```python
from build123d import *

# Parameters (mm, degrees)
BOSS_EXTRU_1_DEPTH      = 3
ESQUISSE2_R             = 17
ENL_V_MAT_EXTRU_1_DEPTH = 3
CONG_1_R                = 10


with BuildPart() as part:
    # Esquisse1 → Boss.-Extru.1 (new body)
    with BuildSketch(Plane.XY):
        Polygon((0, 0), (0, 35), (-3, 35), (-3, 65), (0, 65), (0, 100), (35, 100), (35, 103), (65, 103), (65, 100), (100, 100), (100, 65), (103, 65), (103, 35), (100, 35), (100, 0), (65, 0), (65, -3), (35, -3), (35, 0), align=None)
    extrude(amount=BOSS_EXTRU_1_DEPTH)

    # Esquisse2 → Enlèv. mat.-Extru.1 (cut)
    with BuildSketch(Plane.XY.offset(3)):
        with Locations((50, 50)):
            Circle(ESQUISSE2_R)
    extrude(amount=-ENL_V_MAT_EXTRU_1_DEPTH, mode=Mode.SUBTRACT)

    # Congé1
    cong_1_edges = [part.edges().sort_by_distance(p)[0] for p in [
        (0, 0, 1.5),
        (0, 100, 1.5),
        (100, 100, 1.5),
        (100, 0, 1.5),
    ]]
    fillet(cong_1_edges, radius=CONG_1_R)


solid = part.part
```
Model file for the job. Use its own axes, mm. A direction names the side the tool comes from. Coordinates: 2 decimals unless noted, no trailing zeros. Order: outer loops, then holes, each group sorted by start corner. A loop starts at its lowest first (then second) coordinate and runs counter-clockwise, first axis right, second up. Notation, with made-up numbers: (-25.5, 83.25) -> (-8.5, 83.25) arc R26 ccw to (-8.5, 103.25) -> close; hole circle Ø6 at (25.5, -16.5). An arc over 180 degrees is marked (long way). Answer as a JSON object with one key per item and string values. Group by question number.
1) Which spindle directions (+Z, -Z, +X, -X, +Y, -Y) get a long thin tool onto all of the face, cutting with end or side? Do faces 5 (the face through (65, -1, 1)), 6 (the face through (50, 103, 1)), 7 (the face through (100, 78, 1)), 8 (the face through (35, -2, 1)). Say none if no direction does.
2) Pull direction X, two halves, no side cores. Call faces 1 (the face through (46.315, 33.404, 1.521)), 2 (the face through (2.85, 3.01, 1.52)), 3 (the face through (77, 100, 1)), 4 (the face through (96.99, 97.15, 1.52)): +X half, -X half, draft (parallel to the pull), parting line (faces both ways), or undercut.
3) Cut at D-D, the plane y = 85. Write the cut outline in (x, z), then the cut area to 3 significant figures.
4) Cut at A-A, the plane x = 50. Write the cut outline in (y, z).
5) Drill centre lines: L1, parallel to Y at x = 50, z = 1.9; L2, parallel to Y at x = 42, z = 1; L3, parallel to X at y = 41, z = 2.7. Where is each one in solid material? Low to high.
6) Flat gauge pins, fed straight in: pin 1 (1.5 mm diameter, centred on x = 47.5, y = 34, fed in from -Z); pin 2 (1.5 mm diameter, centred on y = 23, z = 1, fed in from +X); pin 3 (1.5 mm diameter, centred on x = -1, z = 1, fed in from +Y). Where does each tip first touch, or does it go through?
7) Cut at C-C, the plane z = 1.6. Write the cut outline in (x, y).
Check values:
{
 "1": {"face 5": "+Z, -Z, +X, -Y", "face 6": "+Z, -Z, +X, -X, +Y", "face 7": "+Z, -Z, +X, +Y", "face 8": "+Z, -Z, -X, -Y"},
 "2": {"face 1": "undercut", "face 2": "-X half", "face 3": "draft", "face 4": "+X half"},
 "3": {"outline": "(0, 0) -> (100, 0) -> (100, 3) -> (0, 3) -> close", "area": "300 mm²"},
 "4": {"outline": "(-3, 0) -> (33, 0) -> (33, 3) -> (-3, 3) -> close; (67, 0) -> (103, 0) -> (103, 3) -> (67, 3) -> close"},
 "5": {"L1": "y = -3 to 33, 67 to 103", "L2": "y = -3 to 35, 65 to 103", "L3": "x = -3 to 35.58, 64.42 to 103"},
 "6": {"pin 1": "passes through", "pin 2": "stops at x = 100", "pin 3": "stops at y = 65"},
 "7": {"outline": "(-3, 35) -> (0, 35) -> (0, 10) arc R10 ccw to (10, 0) -> (35, 0) -> (35, -3) -> (65, -3) -> (65, 0) -> (90, 0) arc R10 ccw to (100, 10) -> (100, 35) -> (103, 35) -> (103, 65) -> (100, 65) -> (100, 90) arc R10 ccw to (90, 100) -> (65, 100) -> (65, 103) -> (35, 103) -> (35, 100) -> (10, 100) arc R10 ccw to (0, 90) -> (0, 65) -> (-3, 65) -> close; hole circle Ø34 at (50, 50)"}
}
